from build123d import *

# Parameters (mm, degrees)
BOSS_EXTRUDE1_DEPTH      = 30
BOSS_EXTRUDE1_DEPTH_BACK = 30
SKETCH1_R                = 3
CUT_EXTRUDE1_START       = -20
CUT_EXTRUDE1_DEPTH       = 20


with BuildPart() as part:
    # Sketch1 → Boss-Extrude1 (new, two sides: drawn at the far end of the back side and taken through both)
    with BuildSketch(Plane.XY.offset(-BOSS_EXTRUDE1_DEPTH_BACK)):
        with BuildLine():
            Line((-6, 0), (-6, 25))
            Line((-6, 25), (-3, 25))
            Line((-3, 25), (-3, 5.196152423))
            ThreePointArc((-3, 5.196152423), (5.196152423, -3), (-6, 0))
        make_face()
        Circle(SKETCH1_R, mode=Mode.SUBTRACT)
    extrude(amount=BOSS_EXTRUDE1_DEPTH + BOSS_EXTRUDE1_DEPTH_BACK)

    # Sketch2 → Cut-Extrude1 (cut)
    with BuildSketch(Plane.XY.offset(30).offset(CUT_EXTRUDE1_START)):
        with BuildLine():
            Line((-3, 5.196152423), (-6, 5.196152423))
            Line((-6, 5.196152423), (-6, 0))
            ThreePointArc((-6, 0), (5.196152423, -3), (-3, 5.196152423))
        make_face()
    cut_extrude1 = extrude(amount=CUT_EXTRUDE1_DEPTH, mode=Mode.SUBTRACT)

    # Mirror1: Cut-Extrude1 across plane
    add(cut_extrude1.mirror(Plane.XY), mode=Mode.SUBTRACT)


solid = part.part
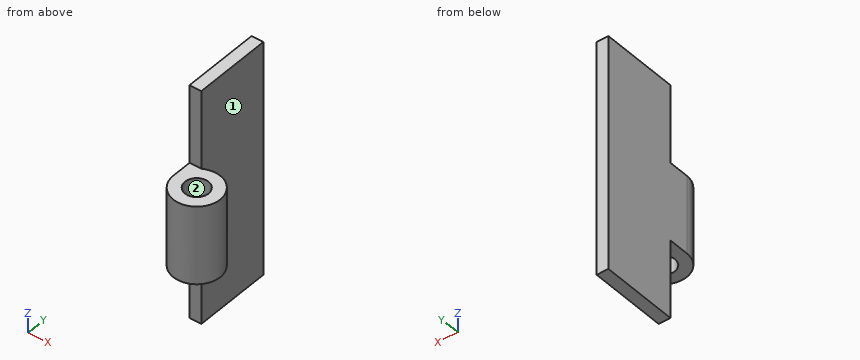
The model under review builds one solid part; all positions refer to its coordinate system, in mm. Face numbers are marked on the shaded views. Round coordinates to 2 decimals unless told otherwise and drop trailing zeros. Loops run counter-clockwise (first coordinate to the right, second up) from the corner with the lowest first, then second, coordinate; pieces in that order, holes last. Notation, with made-up numbers: (49, -10.75) - (79, -10.75) arc R11 ccw to (79, -3.75) - close; hole circle Ø7 at (9.25, 3). An arc over 180 degrees is marked (long way). Use CSV: the item, a comma, the result in double quotes.
(1) Take a section at C-C, the plane y = 21. Give the boundary of the cut face in (x, z).
Working result:
outline,"(-6, -30) - (-3, -30) - (-3, 30) - (-6, 30) - close"
(2) Take a section at D-D, the plane x = -5. Give the boundary of the cut face in (y, z), plus the area to 3 significant figures.
Working result:
outline,"(-3.32, -10) - (5.2, -10) - (5.2, -30) - (25, -30) - (25, 30) - (5.2, 30) - (5.2, 10) - (-3.32, 10) - close"
area,"1,360 mm^2"
(3) For line 1 (Y direction, x = 0, z = 5); line 2 (X direction, y = 19, z = 14); line 3 (Z direction, x = 2.25, y = 5), list the stretches that pass through material, from the lowest coordinate up.
Working result:
line 1,"y = -6 to -3, 3 to 6"
line 2,"x = -6 to -3"
line 3,"z = -10 to 10"
(4) Take a section at A-A, the plane x = 0. Give the boundary of the cut face in (y, z).
Working result:
outline,"(-6, -10) - (-3, -10) - (-3, 10) - (-6, 10) - close; (3, -10) - (6, -10) - (6, 10) - (3, 10) - close"
(5) The part is to be moulded in two halves that separate along Y. For the marked faces 1 and 2, say which applies: pulls with the +Y half, pulls with the -Y half, needs draft (parallel to the pull), parting line crosses it, or undercut.
Working result:
face 1,"needs draft"
face 2,"undercut"
(6) Clearance check with flat-ended pins moving along their axes: P1, Ø3.5, axis at x = -4.5, z = 16.5, coming from the -Y side; P2, Ø6, axis at x = 2, z = 0.5, coming from the +Y side; P3, Ø6, axis at x = 1, y = 0, coming from the -Z side; P4, Ø10, axis at y = 4, z = -14.5, coming from the -X side. State where each tip first meets the part, or that it passes through.
Working result:
P1,"stops at y = 5.2"
P2,"stops at y = 6"
P3,"stops at z = -10"
P4,"stops at x = -6"
(7) Take a section at B-B, the plane z = -9. Give the boundary of the cut face in (x, y).
Working result:
outline,"(-6, 0) arc R6 ccw (long way) to (-3, 5.2) - (-3, 25) - (-6, 25) - close; hole circle Ø6 at (0, 0)"
